Could you check a few things on this model? Use its own coordinates, in mm. A direction names the side the tool comes from. Give positions to 0.01 mm unless a question says otherwise; leave off trailing zeros. Loops run counter-clockwise (first coordinate to the right, second up) from the corner with the lowest first, then second, coordinate; pieces in that order, holes last. Notation, with made-up numbers: M -0.75,70 L 35.25,70 A25 cw 35.25,85 Z; hole C 4,73.25 d4. An arc over 180 degrees is marked long. Use a Markdown table: item, result. Add a question column.
1) Suppose I cut it at B-B on z = 5. List the corners of the cut face in (x, y) for me, and give its area (3 significant figures).
2) Suppose I cut it at A-A on y = -7. List the corners of the cut face in (x, z) for me, and give its area (3 significant figures).
3) If I drill on line 1 along X through (y, z) = (17, 0) (3 decimals); line 2 along X through (y, z) = (30.9, 0); line 3 along Y through (x, z) = (2.75, -4.75), over which ranges is the centre line in solid material (lowest first)? Write a range as [from, to].
4) Which directions (+Z, -Z, +X, -X, +Y, -Y) give clear straight access to the entire face, cutting with the end or side of a thin tool? Please do faces 1 (the flat face through (4.5, 16, 9)), 2 (the flat face through (-1.25, -5.07, 2.21)), 3 (the flat face through (12, 12, 0)), 4 (the flat face through (-12, 12, 0)).
5) Will these pins go through, and if not, where does the flat tip stop? pin 1 Ø1.8 at (x, z) = (12, 0) entering from -Y; pin 2 Ø2.5 at (x, z) = (-10, 0.5) entering from -Y; pin 3 Ø3 at (x, y) = (11, 0) entering from +Z.
6) Suppose I cut it at C-C on z = -8.75. List the corners of the cut face in (x, y) for me, and give its area (3 significant figures).
7) We'd pull the mould along X, two halves only. Please class faces 5 (the flat face through (-12, 6, -1.75)), 6 (the flat face through (0, 16, 4.521)), 7 (the cylindrical face through (3.905, -5.437, -0.867)), 8 (the cylindrical face through (8.75, 5.92, 0.04)): +X half, -X half, draft (parallel to the pull), parting line (faces both ways), or undercut.
```python
from build123d import *

# Parameters (mm, degrees)
SKETCH_1_R          = 14.25
EXTRUDE_1_DEPTH     = 32
SKETCH_3_R          = 1.215
CUT_EXTRUDE_1_DEPTH = 30
SKETCH_4_R          = 4
EXTRUDE_2_DEPTH     = 10
CUT_EXTRUDE_2_DEPTH = 10
CHAMFER_1_SIZE      = 1
SKETCH_6_W          = 9
SKETCH_6_H          = 9
CUT_EXTRUDE_3_DEPTH = 47.58460046
SKETCH_7_R          = 1.15
CUT_EXTRUDE_4_DEPTH = 47.58460046
SKETCH_8_R          = 3
CUT_EXTRUDE_5_DEPTH = 2
CUT_EXTRUDE_6_DEPTH = 12
SKETCH_10_R         = 2.05
CUT_EXTRUDE_7_DEPTH = 29


with BuildPart() as part:
    # Sketch 1 → Extrude 1 (new body)
    with BuildSketch(Plane(origin=(0, 0, 0), x_dir=(1, 0, 0), z_dir=(0, 1, 0))):
        with Locations(Location((0, 0, 0), (0, 0, 270))):
            Circle(SKETCH_1_R)
    extrude(amount=EXTRUDE_1_DEPTH)

    # Sketch 3 → Cut-Extrude 1 (cut)
    with BuildSketch(Plane.XZ):
        with Locations(Location((10.5, 0, 0), (0, 0, 270))):
            Circle(SKETCH_3_R)
        with Locations(Location((-10.5, 0, 0), (0, 0, 90))):
            Circle(SKETCH_3_R)
    extrude(amount=-CUT_EXTRUDE_1_DEPTH, mode=Mode.SUBTRACT)

    # Sketch 4 → Extrude 2 (add)
    with BuildSketch(Plane.XZ):
        with Locations(Location((0, 0, 0), (0, 0, 90))):
            Circle(SKETCH_4_R)
    extrude(amount=EXTRUDE_2_DEPTH)

    # Sketch 5 → Cut-Extrude 2 (cut)
    with BuildSketch(Plane.XZ.offset(10)):
        Polygon((0, -2.932939367), (2.54, -1.466469684), (2.54, 1.466469684), (0, 2.932939367), (-2.54, 1.466469684), (-2.54, -1.466469684), align=None)
    extrude(amount=-CUT_EXTRUDE_2_DEPTH, mode=Mode.SUBTRACT)

    # Chamfer 1
    chamfer_1_edges = [part.edges().sort_by_distance(p)[0] for p in [
        (0, 0, -4),
    ]]
    chamfer(chamfer_1_edges, length=CHAMFER_1_SIZE)

    # Sketch 6 → Cut-Extrude 3 (cut, through all)
    with BuildSketch(Plane(origin=(0, 32, 0), x_dir=(1, 0, 0), z_dir=(0, 1, 0))):
        with Locations((0, -9.020817283)):
            Rectangle(SKETCH_6_W, SKETCH_6_H)
        with BuildLine():
            Line((4.5, -13.520817283), (-4.5, -13.520817283))
            ThreePointArc((-4.5, -13.520817283), (0, -14.25), (4.5, -13.520817283))
        make_face()
    extrude(amount=-CUT_EXTRUDE_3_DEPTH, mode=Mode.SUBTRACT)

    # Sketch 7 → Cut-Extrude 4 (cut, through all)
    with BuildSketch(Plane(origin=(0, 32, 0), x_dir=(1, 0, 0), z_dir=(0, 1, 0))):
        with Locations(Location((-9.969385657, 4.648800879, 0), (0, 0, 270))):
            Circle(SKETCH_7_R)
        with Locations(Location((9.969385657, -4.648800879, 0), (0, 0, 270))):
            Circle(SKETCH_7_R)
    extrude(amount=-CUT_EXTRUDE_4_DEPTH, mode=Mode.SUBTRACT)

    # Sketch 8 → Cut-Extrude 5 (cut)
    with BuildSketch(Plane(origin=(0, 32, 0), x_dir=(1, 0, 0), z_dir=(0, 1, 0))):
        with Locations(Location((0, 0, 0), (0, 0, 270))):
            Circle(SKETCH_8_R)
    extrude(amount=-CUT_EXTRUDE_5_DEPTH, mode=Mode.SUBTRACT)

    # Sketch 9 → Cut-Extrude 6 (cut)
    with BuildSketch(Plane.XZ):
        with BuildLine():
            ThreePointArc((-14.142135624, 1.75), (-14.25, 0), (-14.142135624, -1.75))
            Line((-14.142135624, -1.75), (-10.5, -1.75))
            ThreePointArc((-10.5, -1.75), (-12.25, 0), (-10.5, 1.75))
            Line((-10.5, 1.75), (-14.142135624, 1.75))
        make_face()
        with BuildLine():
            ThreePointArc((-10.5, 1.75), (-12.25, 0), (-10.5, -1.75))
            Line((-10.5, -1.75), (-10.5, -1.215))
            ThreePointArc((-10.5, -1.215), (-11.715, 0), (-10.5, 1.215))
            Line((-10.5, 1.215), (-10.5, 1.75))
        make_face()
        with BuildLine():
            Line((-10.5, -1.215), (-10.5, -1.75))
            ThreePointArc((-10.5, -1.75), (-9.262563133, -1.237436867), (-8.75, 0))
            ThreePointArc((-8.75, 0), (-9.262563133, 1.237436867), (-10.5, 1.75))
            Line((-10.5, 1.75), (-10.5, 1.215))
            ThreePointArc((-10.5, 1.215), (-9.640865261, 0.859134739), (-9.285, 0))
            ThreePointArc((-9.285, 0), (-9.640865261, -0.859134739), (-10.5, -1.215))
        make_face()
        with BuildLine():
            ThreePointArc((10.5, 1.75), (8.75, 0), (10.5, -1.75))
            Line((10.5, -1.75), (10.5, -1.215))
            ThreePointArc((10.5, -1.215), (9.285, 0), (10.5, 1.215))
            Line((10.5, 1.215), (10.5, 1.75))
        make_face()
        with BuildLine():
            Line((10.5, -1.215), (10.5, -1.75))
            ThreePointArc((10.5, -1.75), (11.737436867, -1.237436867), (12.25, 0))
            ThreePointArc((12.25, 0), (11.737436867, 1.237436867), (10.5, 1.75))
            Line((10.5, 1.75), (10.5, 1.215))
            ThreePointArc((10.5, 1.215), (11.359134739, 0.859134739), (11.715, 0))
            ThreePointArc((11.715, 0), (11.359134739, -0.859134739), (10.5, -1.215))
        make_face()
        with BuildLine():
            Line((10.5, -1.75), (14.142135624, -1.75))
            ThreePointArc((14.142135624, -1.75), (14.25, 0), (14.142135624, 1.75))
            Line((14.142135624, 1.75), (10.5, 1.75))
            ThreePointArc((10.5, 1.75), (11.737436867, 1.237436867), (12.25, 0))
            ThreePointArc((12.25, 0), (11.737436867, -1.237436867), (10.5, -1.75))
        make_face()
    extrude(amount=-CUT_EXTRUDE_6_DEPTH, mode=Mode.SUBTRACT)

    # Sketch 10 → Cut-Extrude 7 (cut)
    with BuildSketch(Plane.XZ):
        with Locations(Location((-9.969385657, -4.648800879, 0), (0, 0, 270))):
            Circle(SKETCH_10_R)
        with Locations(Location((9.969385657, 4.648800879, 0), (0, 0, 270))):
            Circle(SKETCH_10_R)
    extrude(amount=-CUT_EXTRUDE_7_DEPTH, mode=Mode.SUBTRACT)


solid = part.part
```
Answer block:
| question | item | result |
|---|---|---|
| 1 | outline | M -13.34,0 L -4.5,0 L -4.5,32 L -13.34,32 Z; M 4.5,0 L 7.95,0 L 7.95,29 L 8.87,29 L 8.87,32 L 4.5,32 Z; M 11.06,29 L 11.99,29 L 11.99,0 L 13.34,0 L 13.34,32 L 11.06,32 Z |
| 1 | area | 442 mm^2 |
| 2 | outline | C 0,0 d8; hole M -2.54,-1.47 L 0,-2.93 L 2.54,-1.47 L 2.54,1.47 L 0,2.93 L -2.54,1.47 Z |
| 2 | area | 27.9 mm^2 |
| 3 | line 1 | x = [-14.25, -11.715], [-9.285, 9.285], [11.715, 14.25] |
| 3 | line 2 | x = [-14.25, -3], [3, 14.25] |
| 3 | line 3 | y = [0, 32] |
| 4 | face 1 | +Z, +Y, -Y |
| 4 | face 2 | -Y |
| 4 | face 3 | +X, -Y |
| 4 | face 4 | -X, -Y |
| 5 | pin 1 | stops at y = 12 |
| 5 | pin 2 | stops at y = 0 |
| 5 | pin 3 | stops at z = 10.62 |
| 6 | outline | M -11.25,0 L 11.25,0 L 11.25,32 L -11.25,32 Z |
| 6 | area | 720 mm^2 |
| 7 | face 5 | draft |
| 7 | face 6 | undercut |
| 7 | face 7 | parting line |
| 7 | face 8 | +X half |
